```python
from build123d import *

# Parameters (mm, degrees)
BOSS_EXTRUDE1_DEPTH = 5
BOSS_EXTRUDE2_DEPTH = 5
FILLET2_R           = 1
FILLET3_R           = 0.2
MIRROR2_START       = -5
MIRROR2_DEPTH       = 10
BOSS_EXTRUDE3_DEPTH = 5
FILLET4_R           = 0.2


# Read off the part's stored shape, not the designer's step: Mirror2
with BuildPart() as part:
    # Sketch1 → Boss-Extrude1 (new, symmetric)
    with BuildSketch(Plane.XY):
        with BuildLine():
            Line((-6, -1), (0, -1))
            Line((0, -1), (0, 1))
            Line((0, 1), (-6, 1))
            Line((-6, 1), (-8, 1))
            Line((-8, 1), (-8, -4))
            ThreePointArc((-8, -4), (-7, -5), (-6, -4))
            Line((-6, -4), (-6, -1))
        make_face()
    extrude(amount=BOSS_EXTRUDE1_DEPTH, both=True)

    # Sketch2 → Boss-Extrude2 (add, symmetric)
    with BuildSketch(Plane.XY):
        with BuildLine():
            Line((-8, -1), (-11, -1))
            ThreePointArc((-11, -1), (-12, 0), (-11, 1))
            Line((-11, 1), (-8, 1))
            ThreePointArc((-8, 1), (-7, 0), (-8, -1))
        make_face()
    extrude(amount=BOSS_EXTRUDE2_DEPTH, both=True)

    # Fillet2
    fillet2_edges = [part.edges().sort_by_distance(p)[0] for p in [
        (-8, -1, 0),
    ]]
    fillet(fillet2_edges, radius=FILLET2_R)

    # Fillet3
    fillet3_edges = [part.edges().sort_by_distance(p)[0] for p in [
        (-6, -1, 0),
    ]]
    fillet(fillet3_edges, radius=FILLET3_R)

    # Mirror2 outline → Mirror2 (add)
    with BuildSketch(Plane.XY.offset(MIRROR2_START)):
        with BuildLine():
            Line((5.8, 1), (0, 1))
            Line((0, 1), (0, -1))
            Line((0, -1), (5.8, -1))
            ThreePointArc((5.8, -1), (5.941421356, -1.058578644), (6, -1.2))
            Line((6, -1.2), (6, -4))
            ThreePointArc((6, -4), (7, -5), (8, -4))
            Line((8, -4), (8, -2))
            ThreePointArc((8, -2), (8.292893219, -1.292893219), (9, -1))
            Line((9, -1), (11, -1))
            ThreePointArc((11, -1), (12, 0), (11, 1))
            Line((11, 1), (9, 1))
            ThreePointArc((9, 1), (8.292893219, 1.292893219), (8, 2))
            Line((8, 2), (8, 4))
            ThreePointArc((8, 4), (7, 5), (6, 4))
            Line((6, 4), (6, 1.2))
            ThreePointArc((6, 1.2), (5.941421356, 1.058578644), (5.8, 1))
        make_face()
        with BuildLine():
            Line((-9, 1), (-5.8, 1))
            ThreePointArc((-5.8, 1), (-5.941421356, 1.058578644), (-6, 1.2))
            Line((-6, 1.2), (-6, 4))
            ThreePointArc((-6, 4), (-7, 5), (-8, 4))
            Line((-8, 4), (-8, 2))
            ThreePointArc((-8, 2), (-8.292893219, 1.292893219), (-9, 1))
        make_face()
    extrude(amount=MIRROR2_DEPTH)

    # Sketch4 → Boss-Extrude3 (add, symmetric)
    with BuildSketch(Plane.XY):
        with BuildLine():
            Line((-6.92611483, 6.197266755), (-0.852229659, 5.747266755))
            ThreePointArc((-0.852229659, 5.747266755), (0.071151926, 4.67611483), (-1, 3.752733245))
            Line((-1, 3.752733245), (-7.07388517, 4.202733245))
            ThreePointArc((-7.07388517, 4.202733245), (-7.997266755, 5.27388517), (-6.92611483, 6.197266755))
        make_face()
        with BuildLine():
            Line((6.057190958, 3.666666667), (5.057190958, 6.495093791))
            ThreePointArc((5.057190958, 6.495093791), (5.666666667, 7.771236166), (6.942809042, 7.161760458))
            Line((6.942809042, 7.161760458), (7.942809042, 4.333333333))
            ThreePointArc((7.942809042, 4.333333333), (7.333333333, 3.057190958), (6.057190958, 3.666666667))
        make_face()
        with BuildLine():
            Line((-6, 5.2), (-6, 4))
            ThreePointArc((-6, 4), (-7, 3), (-8, 4))
            Line((-8, 4), (-8, 5.2))
            ThreePointArc((-8, 5.2), (-7, 6.2), (-6, 5.2))
        make_face()
    extrude(amount=BOSS_EXTRUDE3_DEPTH, both=True)

    # Fillet4
    fillet4_edges = [part.edges().sort_by_distance(p)[0] for p in [
        (-6, 4.123171594, 0),
    ]]
    fillet(fillet4_edges, radius=FILLET4_R)


solid = part.part
```
Check sheet for the modelled part. Datum: model origin and axes. Units: mm. A direction names the side the tool comes from. Round coordinates to 2 decimals unless told otherwise and drop trailing zeros. Write each loop counter-clockwise with the first axis right and the second up, starting at its lowest first coordinate (ties: lowest second). Pieces come first, ordered by that corner, then holes. Notation, with made-up numbers: (59.25, 25) -> (116.25, 25) arc R36 ccw to (116.25, 60) -> close; hole circle Ø7 at (68, 34). An arc over 180 degrees is marked (long way). Put each result on its own line as item: value.
(1) Tool access check on faces 4 (the face through (8, 3, 0)), 5 (the face through (-3.932, 5.975, -0.07)), 6 (the face through (-3.359, 3.928, -0.07)), 7 (the face through (6, -3, 0)). Record the directions out of +Z, -Z, +X, -X, +Y, -Y that give a thin tool (end or side, any length) a straight path to the whole face; none if there is none.
Values found:
face 4: +Z, -Z, +X, +Y
face 5: +Z, -Z, +Y
face 6: +Z, -Z
face 7: +Z, -Z, -Y
(2) Sectioned sample at A-A (y = 2.25). Enter the section's corners in (x, z), plus the area to 3 significant figures.
Values found:
outline: (-8, -5) -> (-6, -5) -> (-6, 5) -> (-8, 5) -> close; (6, -5) -> (8, -5) -> (8, 5) -> (6, 5) -> close
area: 40.0 mm^2
(3) Mould release check, pull along Y, two halves, no side actions. Record for faces 1 (the face through (1, 0, -5)), 2 (the face through (0, 1, 0)), 3 (the face through (-8.301, -1.285, 0.07)): released by +Y, released by -Y, zero draft, split by the parting line, or undercut.
Values found:
face 1: zero draft
face 2: undercut
face 3: released by -Y
(4) Sectioned sample at B-B (x = 10). Enter the section's corners in (y, z), plus the area to 3 significant figures.
Values found:
outline: (-1, -5) -> (1, -5) -> (1, 5) -> (-1, 5) -> close
area: 20.0 mm^2
(5) Go/stop test with flat-tipped pins: pin 1 Ø1 at (y, z) = (4, 0) entering from -X; pin 2 Ø2 at (x, z) = (-10, -1.5) entering from +Y; pin 3 Ø1.5 at (x, z) = (-0.5, 0.5) entering from +Y. Record where each tip stops, or that it passes through.
Values found:
pin 1: stops at x = -8
pin 2: stops at y = 1
pin 3: stops at y = 5.78
(6) Material ranges on line 1 (X direction, y = 3.5, z = -0.75); line 2 (Y direction, x = 4, z = 0.25); line 3 (Y direction, x = -3.75, z = 2.75), recorded low to high.
Values found:
line 1: x = -8 to -6, 6 to 8
line 2: y = -1 to 1
line 3: y = -1 to 1, 3.96 to 5.96
(7) Sectioned sample at C-C (x = 7.25). Enter the section's corners in (y, z).
Values found:
outline: (-4.97, -5) -> (6.29, -5) -> (6.29, 5) -> (-4.97, 5) -> close
